Can you work these out from the model? Positions are in its coordinate system, mm. Face numbers are marked on the shaded views. Give positions to 0.01 mm unless a question says otherwise; leave off trailing zeros. Loops run counter-clockwise (first coordinate to the right, second up) from the corner with the lowest first, then second, coordinate; pieces in that order, holes last. Notation, with made-up numbers: (78.25, -39) - (113.25, -39) arc R20 cw to (113.25, -7) - close; hole circle Ø1 at (13, 10). An arc over 180 degrees is marked (long way). Answer as a JSON object with one key per item and string values.
Autodesk Inventor part; units mm, degrees
ref_plane "YZ Plane" through (0, 0, 0) normal (1, 0, 0) x (0, 1, 0)
ref_plane "XZ Plane" through (0, 0, 0) normal (0, 1, 0) x (-1, 0, 0)
ref_plane "XY Plane" through (0, 0, 0) normal (0, 0, 1) x (1, 0, 0)
sketch "Sketch1" plane through (0, 0, 0) normal (0, 0, 1) x (1, 0, 0)
  line L0 (-3.0081, 0) -> (-3.0081, -1.35)
  line L1 (-0.0086, -1.35) -> (-3.0081, -1.35)
  line L2 (81.9919, -1.35) -> (78.9914, -1.35)
  line L3 (78.9914, -1.35) -> (-0.0086, -1.35)
  line L4 (-3.0081, -1.35) -> (81.9919, -1.35)
  line L5 (81.9919, -1.35) -> (81.9919, -6.35)
  line L6 (81.9919, -6.35) -> (-3.0081, -6.35)
  line L7 (-3.0081, -6.35) -> (-3.0081, -1.35)
  line L8 (0, 12.6) -> (65.5305, 12.6)
  line L9 (0, 0) -> (0, 12.6)
  line L10 (0, 0) -> (3.1074, 0)
  line L11 (3.1074, 0) -> (3.1074, 4.1)
  line L12 (3.1074, 4.1) -> (39.418, 4.1)
  line L13 (39.418, 4.1) -> (39.418, 6.6)
  line L14 (39.418, 6.6) -> (54.418, 6.6)
  line L15 (54.418, 6.6) -> (54.418, 0)
  line L16 (54.418, 0) -> (60.3584, 0)
  line L17 (60.3584, 0) -> (60.3584, 1.0153)
  line L18 (60.3584, 1.0153) -> (65.5305, 1.0153)
  line L19 (65.5305, 1.0153) -> (65.5305, 12.6)
  dimension "d0" = 5
extrude "Extrusion1" add sketch "Sketch1" against normal blind 56.0375 contours L3 L2 L5 L6 L7 L1
fillet "Fillet1" radius 3 4 edges at (-3.0081, -3.85, 0) (-3.0081, -3.85, -56.0375) (81.9919, -3.85, 0) (81.9919, -3.85, -56.0375)
sketch "Sketch2" plane through (0, 0, 0) normal (0, 0, 1) x (1, 0, 0)
  line L0 (0, 12.6) -> (65.5305, 12.6)
  line L1 (0, 0) -> (0, 12.6)
  line L2 (0, 0) -> (3.1074, 0)
  line L3 (3.1074, 0) -> (3.1074, 4.1)
  line L4 (3.1074, 4.1) -> (39.418, 4.1)
  line L5 (39.418, 4.1) -> (39.418, 6.6)
  line L6 (39.418, 6.6) -> (54.418, 6.6)
  line L7 (54.418, 6.6) -> (54.418, 0)
  line L8 (54.418, 0) -> (60.3584, 0)
  line L9 (60.3584, 0) -> (60.3584, 1.0153)
  line L10 (60.3584, 1.0153) -> (65.5305, 1.0153)
  line L11 (65.5305, 1.0153) -> (65.5305, 12.6)
  line L12 (-0.0081, -1.35) -> (78.9919, -1.35)
  line L13 (3.1074, -1.35) -> (54.418, -1.35)
  line L14 (54.418, -1.35) -> (54.418, -4.7625)
  line L15 (54.418, -4.7625) -> (3.1074, -4.7625)
  line L16 (3.1074, -4.7625) -> (3.1074, -1.35)
  line L17 (60.3584, -1.5875) -> (89.6562, -1.5875)
  line L18 (89.6562, -1.5875) -> (89.6562, -4.7625)
  line L19 (89.6562, -4.7625) -> (60.3584, -4.7625)
  line L20 (60.3584, -4.7625) -> (60.3584, -1.5875)
extrude "Extrusion2" cut sketch "Sketch2" against normal blind 56.0375 contours L12 L14 L15 L16 | L17 L18 L19 L20
sketch "Sketch3" plane through (-3.0081, -6.35, -53.0375) normal (-1, 0, 0) x (0, 0, 1)
  line L0 (53.0375, 1.5875) -> (-3, 1.5875)
  line L1 (3.175, 1.5875) -> (46.9313, 1.5875)
  line L2 (46.9313, 1.5875) -> (46.9313, 6.35)
  line L3 (46.9313, 6.35) -> (3.175, 6.35)
  line L4 (3.175, 6.35) -> (3.175, 1.5875)
  point P0 (53.0375, 6.35)
extrude "Extrusion3" cut sketch "Sketch3" against normal blind 89.375
sketch "Sketch4" plane through (0, 0, 0) normal (0, 0, 1) x (1, 0, 0)
  line L0 (60.325, -1.5875) -> (82.55, -1.5875)
  line L1 (82.55, -1.5875) -> (82.55, 0)
  line L2 (82.55, 0) -> (60.325, 0)
  line L3 (60.325, 0) -> (60.325, -1.5875)
  point P0 (0, 0)
extrude "Extrusion4" cut sketch "Sketch4" against normal blind 89.375
properties part number "Heatsink Base" material "Gold"
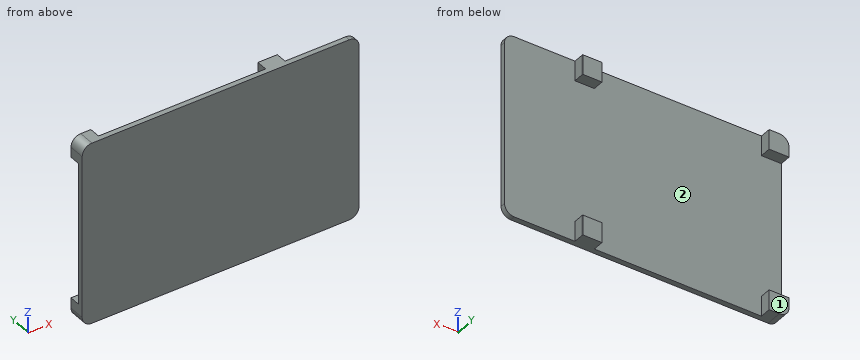
1) If we mould it in two halves opening along X, with no side actions, what happens to the marked faces 1 and 2? For each: released by +X, released by -X, zero draft, split by the parting line, or undercut.
Check sheet entries:
{"face 1": "zero draft", "face 2": "undercut"}
2) I'm going to push flat-ended pins straight in: P1, Ø17, axis at x = 53, z = -21.5, coming from the +Y side; P2, Ø2, axis at y = -3.5, z = -43.5, coming from the -X side; P3, Ø1.7, axis at y = -2.5, z = -3.5, coming from the +X side. Where does each tip first touch, or does it pass through?
Check sheet entries:
{"P1": "y = -4.76", "P2": "through", "P3": "x = 60.36"}
3) I need wall thicknesses on L1, parallel to X at y = -2.25, z = -5; L2, parallel to Y at x = 10, z = -11.5; L3, parallel to Z at x = 55, y = -2.5. Which ranges of each line are inside material? Lowest first, please.
Check sheet entries:
{"L1": "-3.01 to 3.11, 54.42 to 60.36", "L2": "-6.35 to -4.76", "L3": "-56.04 to -49.86, -6.11 to 0"}
4) Imagine slicing it at B-B on x = 57.5. Write out the boundary of the cut face in (y, z), and give its area (3 significant figures).
Check sheet entries:
{"outline": "(-6.35, -56.04) - (-1.35, -56.04) - (-1.35, -49.86) - (-4.76, -49.86) - (-4.76, -6.11) - (-1.35, -6.11) - (-1.35, 0) - (-6.35, 0) - close", "area": "131 mm2"}
5) Imagine slicing it at A-A on y = -3.7. Write out the boundary of the cut face in (x, z).
Check sheet entries:
{"outline": "(-3.01, -53.04) arc R3 ccw to (-0.01, -56.04) - (3.11, -56.04) - (3.11, -49.86) - (-3.01, -49.86) - close; (-3.01, -6.11) - (3.11, -6.11) - (3.11, 0) - (-0.01, 0) arc R3 ccw to (-3.01, -3) - close; (54.42, -56.04) - (60.36, -56.04) - (60.36, -49.86) - (54.42, -49.86) - close; (54.42, -6.11) - (60.36, -6.11) - (60.36, 0) - (54.42, 0) - close"}
6) Imagine slicing it at D-D on x = 10. Write out the boundary of the cut face in (y, z).
Check sheet entries:
{"outline": "(-6.35, -56.04) - (-4.76, -56.04) - (-4.76, 0) - (-6.35, 0) - close"}
